Check sheet for the drawn part. Datum: minimum x, y, z corner. Units: mm. A direction names the side the tool comes from. Round coordinates to 2 decimals unless told otherwise and drop trailing zeros. Write each loop counter-clockwise with the first axis right and the second up, starting at its lowest first coordinate (ties: lowest second). Pieces come first, ordered by that corner, then holes. Notation, with made-up numbers: M 33,48 L 45,48 A28 cw 45,84 Z; hole C 55,84 d5. An arc over 180 degrees is marked long. One line per item, written item: value.
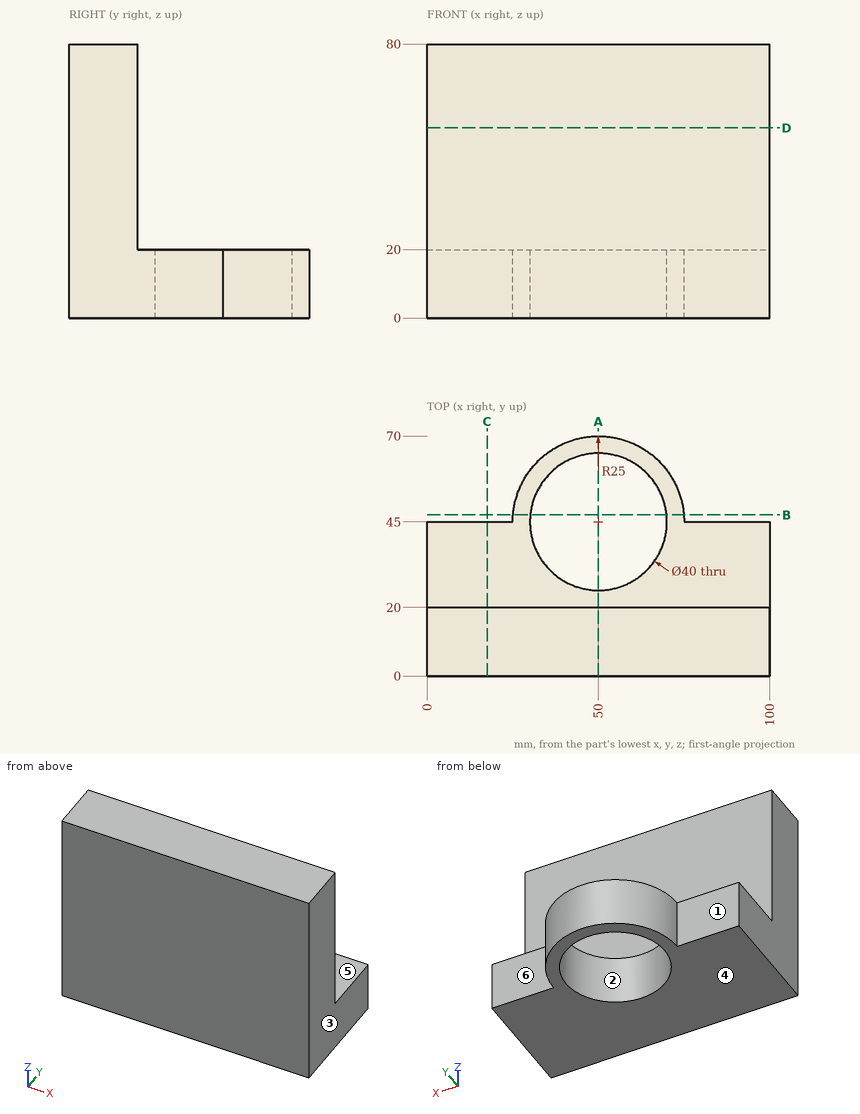
Q1. Depth check by flat-ended pin: P1, Ø1.5, axis at x = 10, y = 44, coming from the +Z side; P2, Ø16, axis at x = 12, z = 14.5, coming from the +Y side; P3, Ø4, axis at x = 27, z = 52, coming from the +Y side. Enter the tip coordinate at first touch or a pass-through.
Completed:
P1: z = 20
P2: y = 45
P3: y = 20
Q2. Sectioned sample at B-B on y = 47. Enter the section's corners in (x, z).
Completed:
outline: M 25.08,0 L 30.1,0 L 30.1,20 L 25.08,20 Z; M 69.9,0 L 74.92,0 L 74.92,20 L 69.9,20 Z
Q3. Scan lines: line 1 (Y direction, x = 50, z = 15); line 2 (Y direction, x = 18.5, z = 46.5); line 3 (Y direction, x = 85.5, z = 17). Record each from-to range of solid material in increasing order. Write a range as [from, to].
Completed:
line 1: [0, 25], [65, 70]
line 2: [0, 20]
line 3: [0, 45]
Q4. Sectioned sample at D-D on z = 55.5. Enter the section's corners in (x, y).
Completed:
outline: M 0,0 L 100,0 L 100,20 L 0,20 Z
Q5. Draft check along X on the marked faces 1, 2 and 3. Enter one of: pulls with the +X half, pulls with the -X half, needs draft (parallel to the pull), parting line crosses it, or undercut.
Completed:
face 1: needs draft
face 2: undercut
face 3: pulls with the +X half
Q6. Sectioned sample at C-C on x = 17.5. Enter the section's corners in (y, z), and give its area (3 significant figures).
Completed:
outline: M 0,0 L 45,0 L 45,20 L 20,20 L 20,80 L 0,80 Z
area: 2,100 mm^2
Q7. Access from +Z, -Z, +X, -X, +Y, -Y to the whole of each face (thin tool, end or side, straight path). Record for the marked faces 4, 5 and 6.
Completed:
face 4: -Z, +X, -X, +Y, -Y
face 5: +Z, +X, -X, +Y
face 6: +Z, -Z, +X, +Y
Q8. Sectioned sample at A-A on x = 50. Enter the section's corners in (y, z), and give its area (3 significant figures).
Completed:
outline: M 0,0 L 25,0 L 25,20 L 20,20 L 20,80 L 0,80 Z; M 65,0 L 70,0 L 70,20 L 65,20 Z
area: 1,800 mm^2
